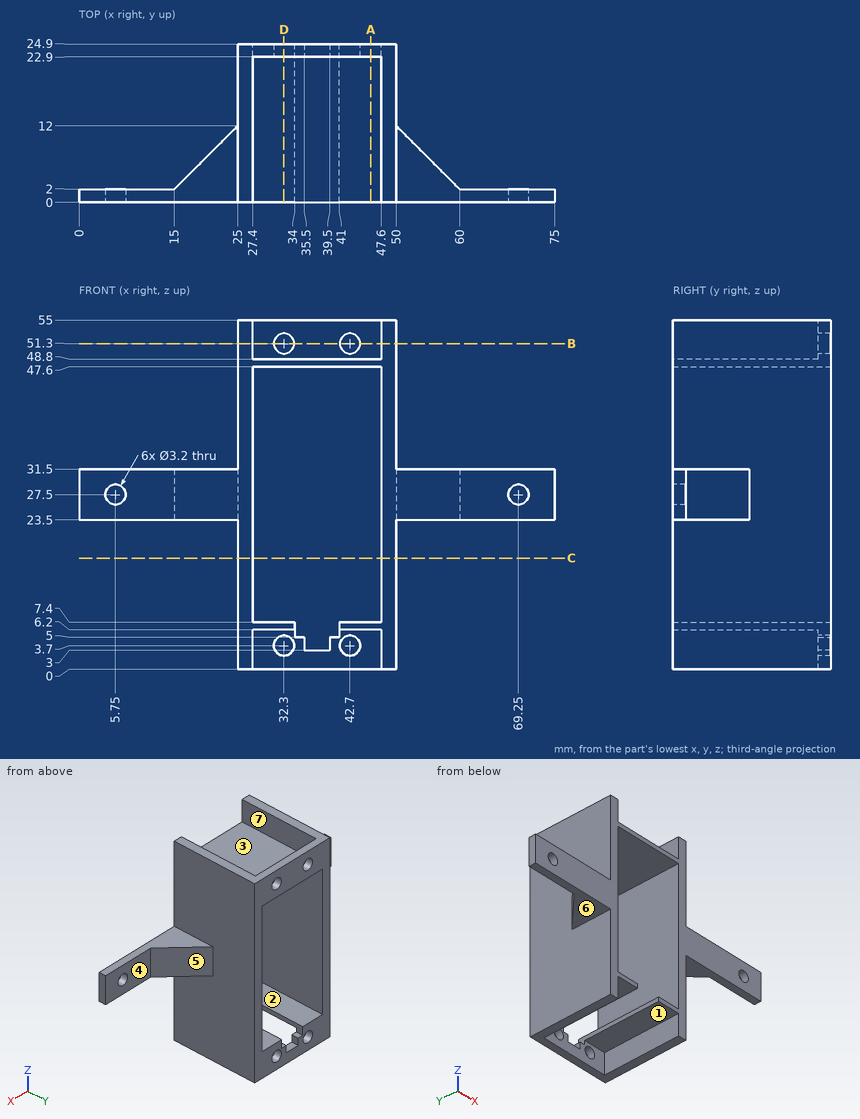
Check sheet for the drawn part. Datum: minimum x, y, z corner. Units: mm. A direction names the side the tool comes from. Coordinates: 2 decimals unless noted, no trailing zeros. Write each loop counter-clockwise with the first axis right and the second up, starting at its lowest first coordinate (ties: lowest second). Pieces come first, ordered by that corner, then holes. Notation, with made-up numbers: M 41,-29.75 L 91,-29.75 A34 cw 91,4.25 Z; hole C -39,-9.5 d4. An arc over 180 degrees is marked long. Use a Markdown table: item, result.
Q1. Sectioned sample at C-C, the plane z = 17.5. Record the boundary of the cut face in (x, y), plus the area to 3 significant figures.
Reply:
| item | result |
|---|---|
| outline | M 25,0 L 27.4,0 L 27.4,24.9 L 25,24.9 Z; M 47.6,0 L 50,0 L 50,24.9 L 47.6,24.9 Z |
| area | 120 mm² |
Q2. Sectioned sample at A-A, the plane x = 46. Record the boundary of the cut face in (y, z).
Reply:
| item | result |
|---|---|
| outline | M 0,6.2 L 22.9,6.2 L 22.9,0 L 24.9,0 L 24.9,7.4 L 0,7.4 Z; M 0,47.6 L 24.9,47.6 L 24.9,55 L 22.9,55 L 22.9,48.8 L 0,48.8 Z |
Q3. Thickness scan on line 1 (Z direction, x = 32.3, y = 23.65); line 2 (X direction, y = 0.6, z = 27.5); line 3 (Z direction, x = 69.25, y = 1.25). Record the ranges inside material, lowest first.
Reply:
| item | result |
|---|---|
| line 1 | z = 0 to 2.1, 5.3 to 7.4, 47.6 to 49.7, 52.9 to 55 |
| line 2 | x = 0 to 4.15, 7.35 to 27.4, 47.6 to 67.65, 70.85 to 75 |
| line 3 | z = 23.5 to 25.9, 29.1 to 31.5 |
Q4. Sectioned sample at B-B, the plane z = 51.3. Record the boundary of the cut face in (x, y).
Reply:
| item | result |
|---|---|
| outline | M 25,0 L 27.4,0 L 27.4,22.9 L 30.7,22.9 L 30.7,24.9 L 25,24.9 Z; M 33.9,22.9 L 41.1,22.9 L 41.1,24.9 L 33.9,24.9 Z; M 44.3,22.9 L 47.6,22.9 L 47.6,0 L 50,0 L 50,24.9 L 44.3,24.9 Z |
Q5. Sectioned sample at D-D, the plane x = 32.3. Record the boundary of the cut face in (y, z).
Reply:
| item | result |
|---|---|
| outline | M 0,6.2 L 22.9,6.2 L 22.9,5.3 L 24.9,5.3 L 24.9,7.4 L 0,7.4 Z; M 0,47.6 L 24.9,47.6 L 24.9,49.7 L 22.9,49.7 L 22.9,48.8 L 0,48.8 Z; M 22.9,0 L 24.9,0 L 24.9,2.1 L 22.9,2.1 Z; M 22.9,52.9 L 24.9,52.9 L 24.9,55 L 22.9,55 Z |
Q6. Set-up check for the marked faces 1, 2, 3 and 4: record each of +Z, -Z, +X, -X, +Y, -Y from which the full face is reachable in a straight line by a thin tool's end or side.
Reply:
| item | result |
|---|---|
| face 1 | -Z, -Y |
| face 2 | +Y, -Y |
| face 3 | +Z, -Y |
| face 4 | +Z, -Z, +X, +Y |
Q7. Draft check along X on the marked faces 5, 6 and 7. Enter one of: +X half, -X half, draft (parallel to the pull), parting line (faces both ways), or undercut.
Reply:
| item | result |
|---|---|
| face 5 | +X half |
| face 6 | draft |
| face 7 | undercut |
Q8. Go/stop test with flat-tipped pins: P1, Ø10, axis at y = 16, z = 9.5, coming from the -X side; P2, Ø3, axis at x = 39, z = 51, coming from the -Y side; P3, Ø5, axis at y = 12.5, z = 51.5, coming from the +X side. Record where each tip stops, or that it passes through.
Reply:
| item | result |
|---|---|
| P1 | stops at x = 25 |
| P2 | stops at y = 22.9 |
| P3 | stops at x = 50 |
